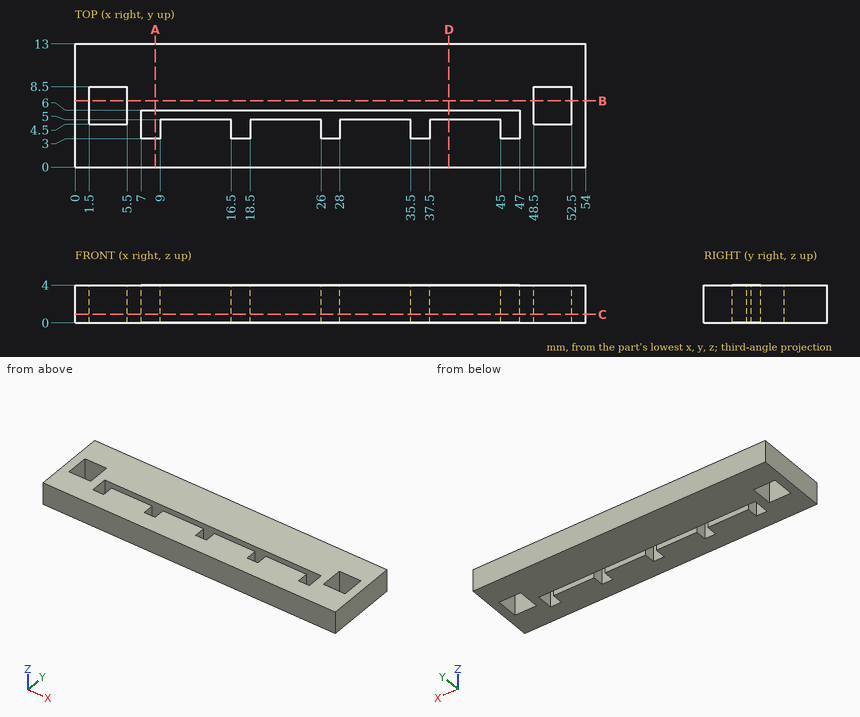
The drawing under review shows one solid part. Ordinate dimensions are in mm from its lowest x, y, z. Give positions to 0.01 mm unless a question says otherwise; leave off trailing zeros. Loops run counter-clockwise (first coordinate to the right, second up) from the corner with the lowest first, then second, coordinate; pieces in that order, holes last. Notation, with made-up numbers: M 66.5,11 L 84.5,11 A35 ccw 84.5,49 Z; hole C -8,-10.75 d1. An arc over 180 degrees is marked long. One line per item, written item: value. Start each with the question number.
Q1. For L1, parallel to X at y = 8.25, z = 3.8; L2, parallel to Y at x = 23.5, z = 3.2; L3, parallel to Y at x = 50, z = 3.6, list the stretches that pass through material, from the lowest coordinate up.
Q2. Add section A-A (x = 8.5). Give the boundary of the cut face in (y, z).
Q3. Add section D-D (x = 39.5). Give the boundary of the cut face in (y, z), and give its area (3 significant figures).
Q4. Clearance check with a flat-ended pin moving along its axis: pin 1 Ø2 at (y, z) = (6.5, 1) entering from -X. State where the tip first meets the part, or that it passes through.
Q5. Add section B-B (y = 7). Give the boundary of the cut face in (x, z).
Q6. Add section C-C (z = 0.9). Count the separate pieces of the cut face and the enclosed holes in it, and give its area (3 significant figures).
Reply:
1. L1: 0 to 1.5, 5.5 to 48.5, 52.5 to 54
1. L2: 0 to 5, 6 to 13
1. L3: 0 to 4.5, 8.5 to 13
2. outline: M 0,0 L 3,0 L 3,4 L 0,4 Z; M 6,0 L 13,0 L 13,4 L 6,4 Z
3. outline: M 0,0 L 5,0 L 5,4 L 0,4 Z; M 6,0 L 13,0 L 13,4 L 6,4 Z
3. area: 48.0 mm²
4. pin 1: x = 0
5. outline: M 0,0 L 1.5,0 L 1.5,4 L 0,4 Z; M 5.5,0 L 48.5,0 L 48.5,4 L 5.5,4 Z; M 52.5,0 L 54,0 L 54,4 L 52.5,4 Z
6. separate pieces: 1
6. enclosed holes: 3
6. area: 610 mm²
